from build123d import *

# Parameters (mm, degrees)
SKETCH_W               = 32
SKETCH_H               = 32
PAD_DEPTH              = 10
SKETCH001_R            = 1.5
PAD001_DEPTH           = 15
SKETCH002_R            = 2
SKETCH002_W            = 15
SKETCH002_H            = 15
PAD002_DEPTH           = 12
PAD002_FACE3_W         = 32
PAD002_FACE3_H         = 10
PAD003_DEPTH           = 256
LINEARPATTERN_COUNT    = 8
LINEARPATTERN_PITCH    = 36.571429
LINEARPATTERN001_COUNT = 8
LINEARPATTERN001_PITCH = 36.571429


with BuildPart() as part:
    # Sketch → Pad (new body)
    with BuildSketch(Plane.XY):
        with Locations((16, 16)):
            Rectangle(SKETCH_W, SKETCH_H)
    extrude(amount=PAD_DEPTH)

    # Sketch001 (on Face6 of Pad) → Pad001 (join)
    with BuildSketch(Plane.XY.offset(10)):
        with Locations((4, 29.5)):
            Circle(SKETCH001_R)
        with Locations((28, 29.5)):
            Circle(SKETCH001_R)
        with Locations((4, 2.5)):
            Circle(SKETCH001_R)
        with Locations((28, 2.5)):
            Circle(SKETCH001_R)
    pad001 = extrude(amount=PAD001_DEPTH)

    # Sketch002 (on Face5 of Pad001) → Pad002 (join)
    with BuildSketch(Plane.XY.offset(10)):
        with Locations((4, 2.5)):
            Circle(SKETCH002_R)
        with Locations((28, 2.5)):
            Circle(SKETCH002_R)
        with Locations((4, 29.5)):
            Circle(SKETCH002_R)
        with Locations((28, 29.5)):
            Circle(SKETCH002_R)
        with Locations((16, 16)):
            Rectangle(SKETCH002_W, SKETCH002_H)
    pad002 = extrude(amount=PAD002_DEPTH)

    # Pad002 Face3 → Pad003 (add)
    with BuildSketch(Plane(origin=(32, 16, 5), x_dir=(0, -1, 0), z_dir=(1, 0, 0))):
        Rectangle(PAD002_FACE3_W, PAD002_FACE3_H)
    extrude(amount=PAD003_DEPTH)

    # LinearPattern: Pad002 ×8
    with Locations(*[(i * LINEARPATTERN_PITCH, 0, 0) for i in range(1, LINEARPATTERN_COUNT)]):
        add(pad002)

    # LinearPattern001: Pad001 ×8
    with Locations(*[(i * LINEARPATTERN001_PITCH, 0, 0) for i in range(1, LINEARPATTERN001_COUNT)]):
        add(pad001)


solid = part.part
The listing builds one solid part. Answer for the finished solid, in the listing's coordinates (mm). A direction names the side the tool comes from. Coordinates: 2 decimals unless noted, no trailing zeros. Loops run counter-clockwise (first coordinate to the right, second up) from the corner with the lowest first, then second, coordinate; pieces in that order, holes last. Notation, with made-up numbers: (63.25, 17) -> (106.25, 17) arc R18 ccw to (106.25, 28) -> close; hole circle Ø8 at (22, 23.5). An arc over 180 degrees is marked (long way). Answer in a Markdown table with one row per item. Add a question column.
1. For faces 1 (the flat face through (60.071, 16, 16)), 2 (the flat face through (16, 23.5, 16)), 3 (the flat face through (235, 8.5, 16)), determine the directions among +Z, -Z, +X, -X, +Y, -Y from which every point of the face is accessible in a straight line to the end or side of a thin tool.
2. Flat-ended cylindrical pins translate along their axes: P1, Ø8, axis at y = 23, z = 15.5, coming from the +X side; P2, Ø4, axis at x = 220, z = 19, coming from the +Y side; P3, Ø12, axis at x = 197.5, y = 18, coming from the +Z side. Find the tip coordinate at first contact, or state that the pin passes through.
3. The part is cut by section A-A, the plane x = 18. Write down the section's boundary in (y, z), then the cut area to 3 significant figures.
4. Consider line 1 (Y direction, x = 206, z = 21); line 2 (Z direction, x = 64, y = 8); line 3 (Z direction, x = 51.5, y = 15). Determine where each line is inside the solid, lowest interval first. Write a range as [from, to].
5. The part is cut by section B-B, the plane z = 19. Count the separate pieces of the cut face and the enclosed holes in it, then the cut area to 3 significant figures.
Answer below:
| question | item | result |
|---|---|---|
| 1 | face 1 | +Z, +Y, -Y |
| 1 | face 2 | +Z, +X, -X, +Y |
| 1 | face 3 | +Z, +X, -X, -Y |
| 2 | P1 | x = 279.5 |
| 2 | P2 | y = 30.9 |
| 2 | P3 | z = 22 |
| 3 | outline | (0, 0) -> (32, 0) -> (32, 10) -> (23.5, 10) -> (23.5, 22) -> (8.5, 22) -> (8.5, 10) -> (0, 10) -> close |
| 3 | area | 500 mm2 |
| 4 | line 1 | [8.5, 23.5] |
| 4 | line 2 | [0, 10] |
| 4 | line 3 | [0, 22] |
| 5 | separate pieces | 40 |
| 5 | enclosed holes | 0 |
| 5 | area | 2,200 mm2 |
